Verification items for the finished model (mm, model axes). Face numbers are marked on the shaded views. A direction names the side the tool comes from. Round coordinates to 2 decimals unless told otherwise and drop trailing zeros. Loops run counter-clockwise (first coordinate to the right, second up) from the corner with the lowest first, then second, coordinate; pieces in that order, holes last. Notation, with made-up numbers: (39.25, 19) - (90.25, 19) arc R10 cw to (90.25, 31) - close; hole circle Ø6 at (41.5, 3.25). An arc over 180 degrees is marked (long way). Use a Markdown table: item, result. Add a question column.
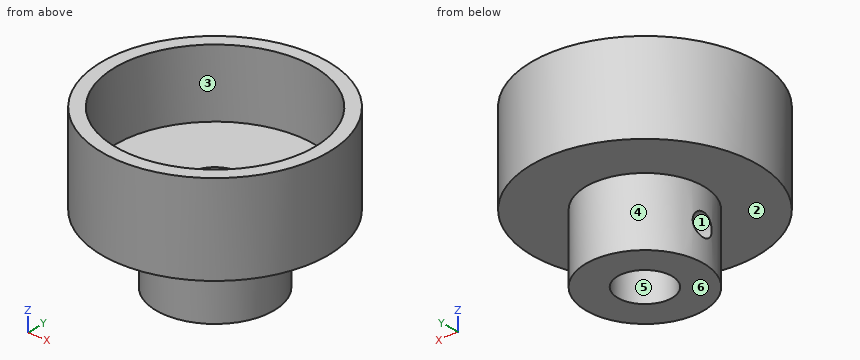
```python
from build123d import *

# Parameters (mm, degrees)
F0_R      = 25
F1_DEPTH  = 20
F2_R      = 13
F3_DEPTH  = 15
F4_R      = 22
F5_DEPTH  = 15
F6_R      = 6
F7_DEPTH  = 35.001
F9_R      = 2.5
F10_DEPTH = 25


with BuildPart() as f1:
    # F0 (on Top) → F1 (new body)
    with BuildSketch(Plane.XY):
        Circle(F0_R)
    extrude(amount=F1_DEPTH)

    # F2 (on face) → F3 (join)
    with BuildSketch(Plane(origin=(0, 0, 0), x_dir=(1, 0, 0), z_dir=(0, 0, -1))):
        Circle(F2_R)
    extrude(amount=F3_DEPTH)

    # F4 (on face) → F5 (cut)
    with BuildSketch(Plane.XY.offset(20)):
        Circle(F4_R)
    extrude(amount=-F5_DEPTH, mode=Mode.SUBTRACT)

    # F6 (on face) → F7 (cut, through all)
    with BuildSketch(Plane(origin=(0, 0, -15), x_dir=(1, 0, 0), z_dir=(0, 0, -1))):
        Circle(F6_R)
    extrude(amount=-F7_DEPTH, mode=Mode.SUBTRACT)

    # F9 (on offset) → F10 (cut)
    with BuildSketch(Plane.YZ.offset(-25)):
        with Locations((0, -7.5)):
            Circle(F9_R)
    extrude(amount=F10_DEPTH, mode=Mode.SUBTRACT)


solid = f1.part
```
Q1. Set-up check for the marked faces 1, 2 and 3: record each of +Z, -Z, +X, -X, +Y, -Y from which the full face is reachable in a straight line by a thin tool's end or side.
Q2. Section check C-C on x = -7. Record the cut outline in (y, z), plus the area to 3 significant figures.
Q3. Release check for a two-part mould opening along Y. For the marked faces 4, 5 and 6 record: +Y half, -Y half, draft (parallel to the pull), parting line (faces both ways), or undercut.
Q4. Go/stop test with flat-tipped pins: pin 1 Ø3 at (y, z) = (0, -7.5) entering from +X; pin 2 Ø12 at (y, z) = (-4.5, 3.5) entering from -X; pin 3 Ø6 at (x, y) = (-2.5, 4.5) entering from +Z; pin 4 Ø10 at (x, z) = (-8.5, -10) entering from -Y. Record where each tip stops, or that it passes through.
Q5. Section check A-A on x = 0. Record the cut outline in (y, z), plus the area to 3 significant figures.
Q6. Section check D-D on y = 18.5. Record the cut outline in (x, z).
Q7. Section check B-B on y = 0. Record the cut outline in (x, z).
Q8. Thickness scan on line 1 along Z through (x, y) = (-10, 0); line 2 along Z through (x, y) = (12, -4.5); line 3 along Z through (x, y) = (10.5, -14.5). Record the ranges inside material, lowest first.
Determined:
| question | item | result |
|---|---|---|
| 1 | face 1 | -X |
| 1 | face 2 | -Z |
| 1 | face 3 | +Z |
| 2 | outline | (-24, 0) - (-10.95, 0) - (-10.95, -15) - (10.95, -15) - (10.95, 0) - (24, 0) - (24, 20) - (20.86, 20) - (20.86, 5) - (-20.86, 5) - (-20.86, 20) - (-24, 20) - close; hole circle Ø5 at (0, -7.5) |
| 2 | area | 643 mm² |
| 3 | face 4 | parting line |
| 3 | face 5 | undercut |
| 3 | face 6 | draft |
| 4 | pin 1 | stops at x = 13 |
| 4 | pin 2 | stops at x = -25 |
| 4 | pin 3 | stops at z = 5 |
| 4 | pin 4 | stops at y = -12.52 |
| 5 | outline | (-25, 0) - (-13, 0) - (-13, -15) - (-6, -15) - (-6, 5) - (-22, 5) - (-22, 20) - (-25, 20) - close; (6, -15) - (13, -15) - (13, 0) - (25, 0) - (25, 20) - (22, 20) - (22, 5) - (6, 5) - close |
| 5 | area | 490 mm² |
| 6 | outline | (-16.82, 0) - (16.82, 0) - (16.82, 20) - (11.91, 20) - (11.91, 5) - (-11.91, 5) - (-11.91, 20) - (-16.82, 20) - close |
| 7 | outline | (-25, 0) - (-13, 0) - (-13, -5) - (-6, -5) - (-6, 5) - (-22, 5) - (-22, 20) - (-25, 20) - close; (-13, -15) - (-6, -15) - (-6, -10) - (-13, -10) - close; (6, -15) - (13, -15) - (13, 0) - (25, 0) - (25, 20) - (22, 20) - (22, 5) - (6, 5) - close |
| 8 | line 1 | z = -15 to -10, -5 to 5 |
| 8 | line 2 | z = -15 to 5 |
| 8 | line 3 | z = 0 to 5 |
